For this review, take the finished solid that the model builds, in its own axes (mm). A direction names the side the tool comes from. Round coordinates to 2 decimals unless told otherwise and drop trailing zeros. Loops run counter-clockwise (first coordinate to the right, second up) from the corner with the lowest first, then second, coordinate; pieces in that order, holes last.
1. Consider section B-B on y = 13.25. State the section outline as (x, z) points, then the cut area to 3 significant figures.
2. To check wall thickness, follow line 1 along Y through (x, z) = (-1.5, 0); line 2 along Y through (x, z) = (-0.5, -3); line 3 along Z through (x, y) = (0.75, 11.75). State the ranges of each line that lie inside material, in increasing order.
3. Consider section A-A on z = 0. State the section outline as (x, y) points.
4. Tool access review of faces 1 (the flat face through (2, 10, 2)), 2 (the flat face through (0, 0, 0)), 3 (the flat face through (-0.81, 12.52, -1.38)): name each direction out of +Z, -Z, +X, -X, +Y, -Y from which nothing blocks a thin tool from reaching the whole face with its end or side.
5. Draft analysis for pull direction Z (two halves, no side actions). For faces 4 (the flat face through (-2, 14, 0)), 5 (the cylindrical face through (0, 5, 2)), 6 (the flat face through (0.81, 12.52, 1.38)), state which applies: released by +Z, released by -Z, zero draft, split by the parting line, or undercut.
6. Consider section D-D on z = 2.5. State the section outline as (x, y) points, then the cut area to 3 significant figures.
7. Clearance check with flat-ended pins moving along their axes: pin 1 Ø1.5 at (y, z) = (12.5, 0.5) entering from +X; pin 2 Ø1.5 at (x, y) = (1.5, 8) entering from +Z; pin 3 Ø4 at (x, y) = (0, 3.5) entering from +Z. State where each tip first meets the part, or that it passes through.
8. Consider section C-C on y = 2. State the section outline as (x, z) points.
Autodesk Inventor part; units mm, degrees
ref_plane "YZ Plane" through (0, 0, 0) normal (1, 0, 0) x (0, 1, 0)
ref_plane "XZ Plane" through (0, 0, 0) normal (0, 1, 0) x (-1, 0, 0)
ref_plane "XY Plane" through (0, 0, 0) normal (0, 0, 1) x (1, 0, 0)
sketch "Sketch1" plane through (0, 0, 0) normal (0, 1, 0) x (-1, 0, 0)
  circle A0 centre (0, 0) radius 2
  dimension "d0" = 4
extrude "Extrusion1" add sketch "Sketch1" along normal blind 10
sketch "Sketch2" plane through (0, 10, 0) normal (0, 1, 0) x (1, 0, 0)
  circle A0 centre (0, 0) radius 2
  circle A1 centre (0, 0) radius 3.5
  dimension "d3" = 7
extrude "Extrusion2" add sketch "Sketch2" along normal blind 4 contours A0 | A1
sketch "Sketch3" plane through (0, 14, 0) normal (0, 1, 0) x (1, 0, 0)
  circle A0 centre (0, 0) radius 3.5
  line L0 (0, 1.8475) -> (1.6, 0.9238)
  line L1 (1.6, 0.9238) -> (1.6, -0.9238)
  line L2 (1.6, -0.9238) -> (0, -1.8475)
  line L3 (0, -1.8475) -> (-1.6, -0.9238)
  line L4 (-1.6, -0.9238) -> (-1.6, 0.9238)
  line L5 (-1.6, 0.9238) -> (0, 1.8475)
  dimension "d6" = 1.6
extrude "Extrusion3" cut sketch "Sketch3" against normal blind 3 contours L0 L1 L2 L3 L4 L5
thread "Thread1"
chamfer "Chamfer1" distance 0.25 angle 45 1 edges at (2, 0, 0)
properties part number "M4x10SHCS"
Resolved:
1. outline: circle Ø7 at (0, 0); hole (-1.6, -0.92) - (0, -1.85) - (1.6, -0.92) - (1.6, 0.92) - (0, 1.85) - (-1.6, 0.92) - close
1. area: 29.6 mm2
2. line 1: y = 0 to 11
2. line 2: y = 10 to 14
2. line 3: z = -3.42 to -1.41, 1.41 to 3.42
3. outline: (-3.5, 10) - (-2, 10) - (-2, 0.25) - (-1.75, 0) - (1.75, 0) - (2, 0.25) - (2, 10) - (3.5, 10) - (3.5, 14) - (1.6, 14) - (1.6, 11) - (-1.6, 11) - (-1.6, 14) - (-3.5, 14) - close
4. face 1: -Y
4. face 2: +Z, -Z, +X, -X, -Y
4. face 3: +Y
5. face 4: zero draft
5. face 5: split by the parting line
5. face 6: undercut
6. outline: (-2.45, 10) - (2.45, 10) - (2.45, 14) - (-2.45, 14) - close
6. area: 19.6 mm2
7. pin 1: stops at x = 3.5
7. pin 2: stops at z = 1.85
7. pin 3: stops at z = 2
8. outline: circle Ø4 at (0, 0)
